Autodesk Inventor part; units mm, degrees
ref_plane "YZ Plane" through (0, 0, 0) normal (1, 0, 0) x (0, 1, 0)
ref_plane "XZ Plane" through (0, 0, 0) normal (0, 1, 0) x (-1, 0, 0)
ref_plane "XY Plane" through (0, 0, 0) normal (0, 0, 1) x (1, 0, 0)
sketch "Sketch1" plane through (0, 0, 0) normal (0, 1, 0) x (-1, 0, 0)
  line L0 (27.1, 36.85) -> (-27.1, 36.85)
  line L1 (-27.1, 36.85) -> (-27.1, -36.85)
  line L2 (-27.1, -36.85) -> (27.1, -36.85)
  line L3 (27.1, -36.85) -> (27.1, 36.85)
  line L4 (37.94, 0) -> (-37.94, 0)
  line L5 (0, -51.59) -> (0, 51.59)
  circle A0 centre (23.5948, 33.3448) radius 1.7526
  circle A1 centre (-23.5952, 33.3448) radius 1.7526
  circle A2 centre (23.5948, -33.3452) radius 1.7526
  circle A3 centre (-23.5952, -33.3452) radius 1.7526
  point P0 (0, 0)
  dimension "d0" = 54.2
  dimension "d1" = 73.7
  dimension "d16" = 3.5052
  dimension "d17" = 3.5052
  dimension "d18" = 3.5052
  dimension "d21" = 47.19
  dimension "d24" = 66.69
extrude "baseplate" add sketch "Sketch1" against normal blind 3.175 contours L3 L4 L5 L0 | L5 L4 L1 L0 | L3 L2 L5 L4 | L5 L2 L1 L4 | A0 | A1 | A2 | A3
sketch "Sketch2" plane through (0, 0, 0) normal (0, 1, 0) x (1, 0, 0)
  line L0 (19, 28.25) -> (-19, 28.25)
  line L1 (-19, 28.25) -> (-19, -28.25)
  line L2 (-19, -28.25) -> (19, -28.25)
  line L3 (19, -28.25) -> (19, 28.25)
  line L4 (-37.94, 0) -> (37.94, 0)
  line L5 (0, 51.59) -> (0, -51.59)
  line L6 (-21, -30.25) -> (-21, 30.25)
  line L7 (-21, 30.25) -> (21, 30.25)
  line L8 (21, 30.25) -> (21, -30.25)
  line L9 (21, -30.25) -> (-21, -30.25)
  dimension "d4" = 38
  dimension "d5" = 56.5
  dimension "d6" = 2
extrude "perimeter" add sketch "Sketch2" along normal blind 10 contours L0 L5 L7 L8 L4 L3 | L0 L1 L4 L6 L7 L5 | L4 L8 L9 L5 L2 L3 | L1 L2 L5 L9 L6 L4
ref_plane "Work Plane1" through (-27.1, 0, 0) normal (0, 0, 1) x (1, 0, 0)
sketch "Sketch3" plane through (-27.1, 0, 0) normal (0, 0, 1) x (1, 0, 0)
  line L0 (48.1, 10) -> (46.1, 10)
  line L1 (46.1, 10) -> (46.1, 19)
  line L2 (46.1, 19) -> (44.1, 19)
  line L3 (48.1, 10) -> (48.1, 23)
  arc A0 (48.1, 23) -> (44.1, 19) centre (48.1, 19) ccw
  line L4 (27.1, 0) -> (27.1, 45.1965)
  line L5 (6.1, 10) -> (8.1, 10)
  line L6 (8.1, 10) -> (8.1, 19)
  line L7 (8.1, 19) -> (10.1, 19)
  line L8 (6.1, 10) -> (6.1, 23)
  arc A1 (10.1, 19) -> (6.1, 23) centre (6.1, 19) ccw
  dimension "d10" = 2
  dimension "d11" = 2
  dimension "d12" = 9
  dimension "d13" = 13
extrude "holders" add sketch "Sketch3" along normal mid plane 26
extrude "Extrusion4" cut sketch "Sketch1" against normal blind 10 contours A0 | A1 | A2 | A3
fillet "Fillet1" radius 5 4 edges at (20, 10, -13) (-20, 10, -13) (20, 10, 13) (-20, 10, 13)
properties part number "esc_holder"
Check sheet for the modelled part. Datum: model origin and axes. Units: mm. A direction names the side the tool comes from. Coordinates: 2 decimals unless noted, no trailing zeros. Loops run counter-clockwise (first coordinate to the right, second up) from the corner with the lowest first, then second, coordinate; pieces in that order, holes last.
1) Sectioned sample at B-B (z = 11). Record the boundary of the cut face in (x, y) (3 decimals).
2) Release check for a two-part mould opening along Z. For faces 1 (the face through (0, 5, -28.25)), 2 (the face through (0, -2, -36.85)), 3 (the face through (20, 12, 14)) record: released by +Z, released by -Z, zero draft, split by the parting line, or undercut.
3) Sectioned sample at A-A (y = 16). Record the boundary of the cut face in (x, z), and give its area (3 significant figures).
4) Gauge pin test, flat ends, axial feed: pin 1 (1 mm diameter, centred on x = -21, z = 14.5, fed in from +Y); pin 2 (3 mm diameter, centred on y = 13, z = 7.5, fed in from +X); pin 3 (2 mm diameter, centred on x = -18.5, y = 18, fed in from +Z). Record the tip position at first contact, or that the pin passes through.
5) Sectioned sample at D-D (y = 8.75). Record the boundary of the cut face in (x, z).
6) Sectioned sample at C-C (x = -10). Record the boundary of the cut face in (y, z) (3 decimals).
7) Access from +Z, -Z, +X, -X, +Y, -Y to the whole of each face (thin tool, end or side, straight path). Record for faces 4 (the face through (-21, 9, 0)), 5 (the face through (21, 9, 0)), 6 (the face through (-19.5, 19.1, -13)).
8) Material ranges on probe 1 along X at (y, z) = (6.25, -6); probe 2 along Z at (x, y) = (15, 6.75); probe 3 along Z at (x, y) = (22.5, -1.5), recorded low to high.
Check sheet entries:
1. outline: (-27.1, -3.175) - (27.1, -3.175) - (27.1, 0) - (21, 0) - (21, 23) arc R4 ccw to (17, 19) - (19, 19) - (19, 0) - (-19, 0) - (-19, 19) - (-17, 19) arc R4 ccw to (-21, 23) - (-21, 0) - (-27.1, 0) - close
2. face 1: undercut
2. face 2: released by -Z
2. face 3: released by +Z
3. outline: (-21, -13) - (-19, -13) - (-19, 13) - (-21, 13) - close; (19, -13) - (21, -13) - (21, 13) - (19, 13) - close
3. area: 104 mm2
4. pin 1: stops at y = 12
4. pin 2: stops at x = 21
4. pin 3: stops at z = 13
5. outline: (-21, -30.25) - (21, -30.25) - (21, 30.25) - (-21, 30.25) - close; hole (-19, -28.25) - (19, -28.25) - (19, 28.25) - (-19, 28.25) - close
6. outline: (-3.175, -36.85) - (0, -36.85) - (0, -30.25) - (10, -30.25) - (10, -28.25) - (0, -28.25) - (0, 28.25) - (10, 28.25) - (10, 30.25) - (0, 30.25) - (0, 36.85) - (-3.175, 36.85) - close
7. face 4: +Z, -Z, -X, +Y
7. face 5: +Z, -Z, +X, +Y
7. face 6: -Z, +X, -X, +Y
8. probe 1: x = -21 to -19, 19 to 21
8. probe 2: z = -30.25 to -28.25, 28.25 to 30.25
8. probe 3: z = -36.85 to -34.71, -31.98 to 31.98, 34.71 to 36.85
